Part print with two shaded views. Sizes in mm from the minimum x, y, z corner. Give positions to 0.01 mm unless a question says otherwise; leave off trailing zeros. Order: outer loops, then holes, each group sorted by start corner. A loop starts at its lowest first (then second) coordinate and runs counter-clockwise, first axis right, second up. Notation, with made-up numbers: (27, 15.5) - (31, 15.5) arc R25 ccw to (31, 32.5) - close; hole circle Ø3 at (28.25, -10.75). An arc over 180 degrees is marked (long way). Return JSON: item names as keys, results as strings. Group by question number.
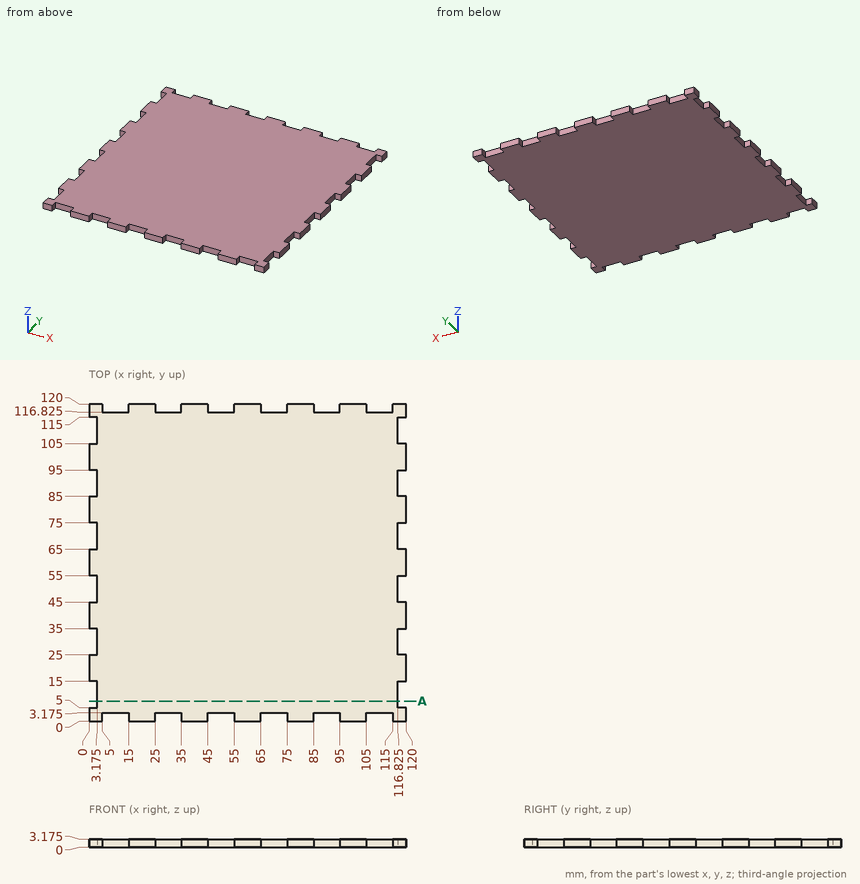
(1) Drill centre line: L1, parallel to Y at x = 34.5, z = 1.95 (3 decimals). Where is it in solid material? Low to high.
(2) Slice it at A-A (y = 7.5). Give the cut face in (x, z) (3 decimals).
(3) Drop flat-ended pins along their axis: pin 1 Ø1.6 at (x, z) = (2, 1) entering from -Y; pin 2 Ø1 at (y, z) = (92.5, 2.5) entering from -X (3 decimals); pin 3 Ø1.5 at (y, z) = (69, 2) entering from +X (3 decimals). Give the stop position or say it passes through.
Result set:
{
 "1": {"L1": "y = 3.175 to 116.825"},
 "2": {"outline": "(3.175, 0) - (116.825, 0) - (116.825, 3.175) - (3.175, 3.175) - close"},
 "3": {"pin 1": "stops at y = 0", "pin 2": "stops at x = 3.175", "pin 3": "stops at x = 116.825"}
}
